```python
from build123d import *

# Parameters (mm, degrees)
SKETCH_1_R      = 0.75
SKETCH_1_R_2    = 2
EXTRUDE_1_DEPTH = 8
SKETCH_2_R      = 10
SKETCH_2_R_2    = 1
EXTRUDE_2_DEPTH = 10


with BuildPart() as part:
    # 草圖1 → 填料-伸長1 (new body)
    with BuildSketch(Plane(origin=(0, 0, 0), x_dir=(1, 0, 0), z_dir=(0, 1, 0))):
        with BuildLine():
            Line((-0.414012206, -4), (25, -4))
            Line((25, -4), (34, -4))
            ThreePointArc((34, -4), (38, 0), (34, 4))
            Line((34, 4), (25, 4))
            Line((25, 4), (-0.414012206, 4))
            Line((-0.414012206, 4), (-34, 4))
            ThreePointArc((-34, 4), (-38, 0), (-34, -4))
            Line((-34, -4), (-0.414012206, -4))
        make_face()
        with Locations(Location((34, 0, 0), (0, 0, 270))):
            Circle(SKETCH_1_R, mode=Mode.SUBTRACT)
        with Locations(Location((-34, 0, 0), (0, 0, 270))):
            Circle(SKETCH_1_R, mode=Mode.SUBTRACT)
        with Locations(Location((-25, 0, 0), (0, 0, 270))):
            Circle(SKETCH_1_R_2, mode=Mode.SUBTRACT)
        with Locations(Location((25, 0, 0), (0, 0, 270))):
            Circle(SKETCH_1_R_2, mode=Mode.SUBTRACT)
        with Locations(Location((-16, 0, 0), (0, 0, 270))):
            Circle(SKETCH_1_R, mode=Mode.SUBTRACT)
        with Locations(Location((16, 0, 0), (0, 0, 270))):
            Circle(SKETCH_1_R, mode=Mode.SUBTRACT)
    extrude(amount=EXTRUDE_1_DEPTH)

    # 草圖2 → 填料-伸長2 (add)
    with BuildSketch(Plane(origin=(0, 8, 0), x_dir=(-1, 0, 0), z_dir=(0, 1, 0))):
        with Locations(Location((0, 0, 0), (0, 0, 90))):
            Circle(SKETCH_2_R)
        with Locations(Location((0, -4, 0), (0, 0, 90))):
            Circle(SKETCH_2_R_2, mode=Mode.SUBTRACT)
        with Locations(Location((0, 4, 0), (0, 0, 90))):
            Circle(SKETCH_2_R_2, mode=Mode.SUBTRACT)
    extrude(amount=-EXTRUDE_2_DEPTH)


solid = part.part
```
Here's how the part is built. I have some questions about the finished solid (model axes, mm). A direction names the side the tool comes from. Round coordinates to 2 decimals unless told otherwise and drop trailing zeros. Loops run counter-clockwise (first coordinate to the right, second up) from the corner with the lowest first, then second, coordinate; pieces in that order, holes last. Notation, with made-up numbers: (56, 49.5) -> (95, 49.5) arc R13 ccw to (95, 61.5) -> close; hole circle Ø9 at (-16, 65). An arc over 180 degrees is marked (long way). Answer as CSV lines item,"result". Start each with the question number.
1. Imagine slicing it at D-D on x = 25. Write out the boundary of the cut face in (y, z), plus the area to 3 significant figures.
2. Imagine slicing it at B-B on y = 5.25. State how many separate pieces and enclosed holes the cut face has, plus the area to 3 significant figures.
3. For faces 4 (the face through (21, 4, 4)), 5 (the face through (-21, 4, -4)), 6 (the face through (-22, 4, 4)), 7 (the face through (0, 4, 4)), which set-ups out of +Z, -Z, +X, -X, +Y, -Y let a thin tool reach every point of the face, with its end or its side?
4. Imagine slicing it at A-A on x = -16. Write out the boundary of the cut face in (y, z), plus the area to 3 significant figures.
5. If we mould it in two halves opening along X, with no side actions, what happens to faces 1 (the face through (23, 0, -2)), 2 (the face through (-26.2, 3.9, -1.6)), 3 (the face through (-38, 4, 0))? For each: pulls with the +X half, pulls with the -X half, needs draft (parallel to the pull), parting line crosses it, or undercut.
6. I'm going to push flat-ended pins straight in: P1, Ø2.5, axis at x = 20, y = 2, coming from the +Z side; P2, Ø1.5, axis at y = 4, z = -7, coming from the +X side; P3, Ø4, axis at x = 26.5, y = 5, coming from the -Z side. Where does each tip first touch, or does it pass through?
7. I need wall thicknesses on probe 1 along Y at (x, z) = (23, -3.75); probe 2 along Z at (x, y) = (22.5, 2.5); probe 3 along X at (y, z) = (-1.5, 6). Which ranges of each line are inside material? Lowest first, please. Write a range as from..to.
Solution:
1,outline,"(0, -4) -> (8, -4) -> (8, -2) -> (0, -2) -> close; (0, 2) -> (8, 2) -> (8, 4) -> (0, 4) -> close"
1,area,"32.0 mm²"
2,separate pieces,"1"
2,enclosed holes,"8"
2,area,"717 mm²"
3,face 4,"+Z, +X, +Y, -Y"
3,face 5,"-Z, -X, +Y, -Y"
3,face 6,"+Z, -X, +Y, -Y"
3,face 7,"+Y, -Y"
4,outline,"(0, -4) -> (8, -4) -> (8, -0.75) -> (0, -0.75) -> close; (0, 0.75) -> (8, 0.75) -> (8, 4) -> (0, 4) -> close"
4,area,"52.0 mm²"
5,face 1,"needs draft"
5,face 2,"undercut"
5,face 3,"pulls with the -X half"
6,P1,"z = 4"
6,P2,"x = 7.81"
6,P3,"z = -4"
7,probe 1,"0..8"
7,probe 2,"-4..4"
7,probe 3,"-8..8"
